Read the model definition and answer for the solid it produces. Units are mm, in the model's axes. Face numbers are marked on the shaded views. Coordinates: 2 decimals unless noted, no trailing zeros. Order: outer loops, then holes, each group sorted by start corner. A loop starts at its lowest first (then second) coordinate and runs counter-clockwise, first axis right, second up. Notation, with made-up numbers: (7, 12.5) - (14, 12.5) arc R24 cw to (14, 42.5) - close; hole circle Ø5 at (67, 42.25). An arc over 180 degrees is marked (long way). Write item = value, one per line.
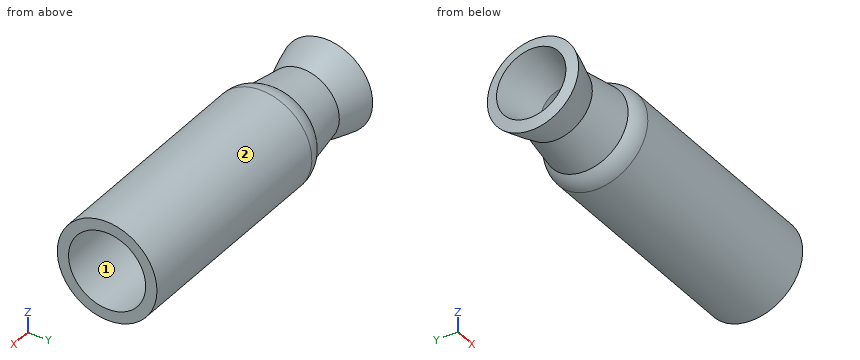
from build123d import *


with BuildPart() as part:
    # Sketch1 → Revolve1 (revolve)
    with BuildSketch(Plane.XY, mode=Mode.PRIVATE) as revolve1_sk:
        with BuildLine():
            Line((28.949236933, 27.386004017), (189.133015331, 27.386004017))
            Line((189.133015331, 27.386004017), (189.133015331, 35.386004017))
            Line((189.133015331, 35.386004017), (28.949236933, 35.386004017))
            ThreePointArc((28.949236933, 35.386004017), (22.060935151, 34.015835602), (16.221314872, 30.113926078))
            Line((16.221314872, 30.113926078), (7.884849119, 21.777460326))
            ThreePointArc((7.884849119, 21.777460326), (5.344435892, 20.007381854), (2.348184674, 19.226769399))
            add(Edge.make_bspline(
                [(2.348184674, 19.226769399), (0.313545637, 20.077506038), (-5.800272608, 22.518234312), (-11.933859147, 24.735791909), (-13.981586932, 25.43765231)],
                knots=[0.018493807, 0.018493807, 0.018493807, 0.117487589, 0.315475154, 0.414468937, 0.414468937, 0.414468937], degree=2))
            add(Edge.make_bspline(
                [(-13.981586932, 25.43765231), (-16.029314717, 26.139512711), (-28.160190771, 30.070121673), (-38.315022829, 32.432092239)],
                knots=[0.414468937, 0.414468937, 0.414468937, 0.513462719, 1, 1, 1], degree=2))
            Line((-38.315022829, 32.432092239), (-40.127010283, 24.64))
            add(Edge.make_bspline(
                [(-8.337690555, 14.885570905), (-24.160193055, 20.927046968), (-40.127010283, 24.64)],
                knots=[0.208731219, 0.208731219, 0.208731219, 1, 1, 1], degree=2))
            ThreePointArc((-8.337690555, 14.885570905), (2.839826237, 16.044626201), (13.541703369, 19.472470519))
            ThreePointArc((13.541703369, 19.472470519), (16.609976492, 20.839222591), (19.662309445, 22.241212152))
            Line((19.662309445, 22.241212152), (21.878169121, 24.457071829))
            ThreePointArc((21.878169121, 24.457071829), (25.12240261, 26.624799342), (28.949236933, 27.386004017))
        make_face()
        with BuildLine():
            Line((7.884849119, 21.777460326), (16.221314872, 30.113926078))
            Line((16.221314872, 30.113926078), (-13.981586932, 25.43765231))
            add(Edge.make_bspline(
                [(2.348184674, 19.226769399), (0.313545637, 20.077506038), (-5.800272608, 22.518234312), (-11.933859147, 24.735791909), (-13.981586932, 25.43765231)],
                knots=[0.018493807, 0.018493807, 0.018493807, 0.117487589, 0.315475154, 0.414468937, 0.414468937, 0.414468937], degree=2))
            ThreePointArc((2.348184674, 19.226769399), (5.344435892, 20.007381854), (7.884849119, 21.777460326))
        make_face()
    revolve(revolve1_sk.sketch.rotate(Axis((0, 0, 0), (-1, 0, 0)), 90), axis=Axis((0, 0, 0), (-1, 0, 0)))


solid = part.part
1) The part is cut by section A-A (x = 84.5). Determine the outline of the cut face in (y, z).
Returned:
outline = circle Ø70.77 at (0, 0); hole circle Ø54.77 at (0, 0)
2) Straight lines are drawn through the part: line 1 along Y through (x, z) = (87, 0); line 2 along Y through (x, z) = (92.5, 1.5); line 3 along Z through (x, y) = (49, -19.5). For each, find the intervals that lie inside material, in ascending order. Write a range as from..to.
Returned:
line_1 = -35.39..-27.39, 27.39..35.39
line_2 = -35.35..-27.34, 27.34..35.35
line_3 = -29.53..-19.23, 19.23..29.53
3) Flat-ended cylindrical pins translate along their axes: pin 1 Ø10 at (x, z) = (57, -28) entering from -Y; pin 2 Ø1.5 at (x, z) = (-13, -6.5) entering from -Y; pin 3 Ø8 at (x, z) = (25.5, -2.5) entering from -Y. Find the tip coordinate at first contact, or state that the pin passes through.
Returned:
pin_1 = -26.89
pin_2 = -24.97
pin_3 = -35.38
4) Determine the mould class of the marked faces 1 and 2 for opening direction Y: pulls with the +Y half, pulls with the -Y half, needs draft (parallel to the pull), parting line crosses it, or undercut.
Returned:
face_1 = undercut
face_2 = parting line crosses it
